```python
from build123d import *

# Parameters (mm, degrees)
F0_R     = 6
F1_DEPTH = 3.7
F2_R     = 1.44999
F4_DEPTH = 14
F5_R     = 1


# Not quite as in the source:
# - a fillet or chamfer is up to 0.001 mm smaller than in the source, because OpenCascade refuses the exact size


with BuildPart() as f1:
    # F0 (on Top) → F1 (new body)
    with BuildSketch(Plane.XY):
        with BuildLine():
            ThreePointArc((6.8481749394, -1.45), (6.9619402675, -0.7289634506), (7, 0))
            ThreePointArc((7, 0), (6.9619402675, 0.7289634506), (6.8481749394, 1.45))
            ThreePointArc((6.8481749394, 1.45), (4.9497474683, 4.9497474683), (1.45, 6.8481749394))
            ThreePointArc((1.45, 6.8481749394), (0.7289634506, 6.9619402675), (0, 7))
            ThreePointArc((0, 7), (-0.7289634506, 6.9619402675), (-1.45, 6.8481749394))
            ThreePointArc((-1.45, 6.8481749394), (-4.9497474683, 4.9497474683), (-6.8481749394, 1.45))
            ThreePointArc((-6.8481749394, 1.45), (-6.9619402675, 0.7289634506), (-7, 0))
            ThreePointArc((-7, 0), (-6.9619402675, -0.7289634506), (-6.8481749394, -1.45))
            ThreePointArc((-6.8481749394, -1.45), (-4.9497474683, -4.9497474683), (-1.45, -6.8481749394))
            ThreePointArc((-1.45, -6.8481749394), (-0.7289634506, -6.9619402675), (0, -7))
            ThreePointArc((0, -7), (0.7289634506, -6.9619402675), (1.45, -6.8481749394))
            ThreePointArc((1.45, -6.8481749394), (4.9497474683, -4.9497474683), (6.8481749394, -1.45))
        make_face()
        Circle(F0_R, mode=Mode.SUBTRACT)
        with BuildLine():
            Line((23.2, 0), (7, 0))
            ThreePointArc((7, 0), (6.9619402675, -0.7289634506), (6.8481749394, -1.45))
            Line((6.8481749394, -1.45), (23.2, -1.45))
            Line((23.2, -1.45), (23.2, 0))
        make_face()
        with BuildLine():
            ThreePointArc((6.8481749394, 1.45), (6.9619402675, 0.7289634506), (7, 0))
            Line((7, 0), (23.2, 0))
            Line((23.2, 0), (23.2, 1.45))
            Line((23.2, 1.45), (6.8481749394, 1.45))
        make_face()
        with BuildLine():
            ThreePointArc((0, 7), (0.7289634506, 6.9619402675), (1.45, 6.8481749394))
            Line((1.45, 6.8481749394), (1.45, 23.2))
            Line((1.45, 23.2), (0, 23.2))
            Line((0, 23.2), (0, 7))
        make_face()
        with BuildLine():
            Line((1.45, -23.2), (1.45, -6.8481749394))
            ThreePointArc((1.45, -6.8481749394), (0.7289634506, -6.9619402675), (0, -7))
            Line((0, -7), (0, -23.2))
            Line((0, -23.2), (1.45, -23.2))
        make_face()
        with BuildLine():
            ThreePointArc((-1.45, 6.8481749394), (-0.7289634506, 6.9619402675), (0, 7))
            Line((0, 7), (0, 23.2))
            Line((0, 23.2), (-1.45, 23.2))
            Line((-1.45, 23.2), (-1.45, 6.8481749394))
        make_face()
        with BuildLine():
            Line((0, -23.2), (0, -7))
            ThreePointArc((0, -7), (-0.7289634506, -6.9619402675), (-1.45, -6.8481749394))
            Line((-1.45, -6.8481749394), (-1.45, -23.2))
            Line((-1.45, -23.2), (0, -23.2))
        make_face()
        with BuildLine():
            ThreePointArc((-7, 0), (-6.9619402675, 0.7289634506), (-6.8481749394, 1.45))
            Line((-6.8481749394, 1.45), (-23.2, 1.45))
            Line((-23.2, 1.45), (-23.2, 0))
            Line((-23.2, 0), (-7, 0))
        make_face()
        with BuildLine():
            Line((-23.2, -1.45), (-6.8481749394, -1.45))
            ThreePointArc((-6.8481749394, -1.45), (-6.9619402675, -0.7289634506), (-7, 0))
            Line((-7, 0), (-23.2, 0))
            Line((-23.2, 0), (-23.2, -1.45))
        make_face()
    extrude(amount=F1_DEPTH)

    # F2 (radius 1.45 in the source; OpenCascade refuses exactly that, so slightly less here)
    f2_edges = [f1.edges().sort_by_distance(p)[0] for p in [
        (1.45, 15.024087, 0),
        (15.024087, 1.45, 0),
        (15.024087, -1.45, 0),
        (1.45, -15.024087, 0),
        (-1.45, -15.024087, 0),
        (-15.024087, -1.45, 0),
        (-15.024087, 1.45, 0),
        (-1.45, 15.024087, 0),
    ]]
    fillet(f2_edges, radius=F2_R)

    # F3 (on face) → F4 (join)
    with BuildSketch(Plane.XY.offset(3.7)):
        with BuildLine():
            Line((18.4430881362, 1.45), (18.4430881362, -1.45))
            ThreePointArc((18.4430881362, -1.45), (18.5, 0), (18.4430881362, 1.45))
        make_face()
        with BuildLine():
            Line((6.8481749394, -1.45), (18.4430881362, -1.45))
            Line((18.4430881362, -1.45), (18.4430881362, 1.45))
            Line((18.4430881362, 1.45), (6.8481749394, 1.45))
            ThreePointArc((6.8481749394, 1.45), (7, 0), (6.8481749394, -1.45))
        make_face()
        with BuildLine():
            ThreePointArc((-18.4430881362, 1.45), (-18.5, 0), (-18.4430881362, -1.45))
            Line((-18.4430881362, -1.45), (-18.4430881362, 1.45))
        make_face()
        with BuildLine():
            Line((-18.4430881362, 1.45), (-18.4430881362, -1.45))
            Line((-18.4430881362, -1.45), (-6.8481749394, -1.45))
            ThreePointArc((-6.8481749394, -1.45), (-7, 0), (-6.8481749394, 1.45))
            Line((-6.8481749394, 1.45), (-18.4430881362, 1.45))
        make_face()
        with BuildLine():
            ThreePointArc((-1.45, -18.4430881362), (0, -18.5), (1.45, -18.4430881362))
            Line((1.45, -18.4430881362), (-1.45, -18.4430881362))
        make_face()
        with BuildLine():
            Line((-1.45, -18.4430881362), (1.45, -18.4430881362))
            Line((1.45, -18.4430881362), (1.45, -6.8481749394))
            ThreePointArc((1.45, -6.8481749394), (0, -7), (-1.45, -6.8481749394))
            Line((-1.45, -6.8481749394), (-1.45, -18.4430881362))
        make_face()
        with BuildLine():
            Line((1.45, 6.8481749394), (1.45, 18.4430881362))
            Line((1.45, 18.4430881362), (-1.45, 18.4430881362))
            Line((-1.45, 18.4430881362), (-1.45, 6.8481749394))
            ThreePointArc((-1.45, 6.8481749394), (0, 7), (1.45, 6.8481749394))
        make_face()
        with BuildLine():
            Line((-1.45, 18.4430881362), (1.45, 18.4430881362))
            ThreePointArc((1.45, 18.4430881362), (0, 18.5), (-1.45, 18.4430881362))
        make_face()
    extrude(amount=F4_DEPTH)

    # F5
    f5_edges = [f1.edges().sort_by_distance(p)[0] for p in [
        (12.645632, 1.45, 17.7),
        (18.443088, 1.45, 10.7),
        (20.821544, 1.45, 3.7),
        (20.821544, -1.45, 3.7),
        (18.443088, -1.45, 10.7),
        (12.645632, -1.45, 17.7),
        (1.45, 12.645632, 17.7),
        (-1.45, 12.645632, 17.7),
        (1.45, 18.443088, 10.7),
        (-1.45, 18.443088, 10.7),
        (1.45, 20.821544, 3.7),
        (-1.45, 20.821544, 3.7),
        (0, 18.5, 3.7),
        (-18.443088, 1.45, 10.7),
        (-18.443088, -1.45, 10.7),
        (-20.821544, 1.45, 3.7),
        (-1.45, -18.443088, 10.7),
        (1.45, -18.443088, 10.7),
        (-1.45, -20.821544, 3.7),
        (1.45, -20.821544, 3.7),
        (-20.821544, -1.45, 3.7),
        (-12.645632, 1.45, 17.7),
        (-12.645632, -1.45, 17.7),
        (-1.45, -12.645632, 17.7),
        (1.45, -12.645632, 17.7),
        (-1.45, -6.848175, 10.7),
        (1.45, -6.848175, 10.7),
        (6.848175, -1.45, 10.7),
        (6.848175, 1.45, 10.7),
        (1.45, 6.848175, 10.7),
        (-1.45, 6.848175, 10.7),
        (-6.848175, 1.45, 10.7),
        (-6.848175, -1.45, 10.7),
    ]]
    fillet(f5_edges, radius=F5_R)


solid = f1.part
```
Geometry check sheet. Reference: the model listing, model coordinates, mm. A direction names the side the tool comes from. Round coordinates to 2 decimals unless told otherwise and drop trailing zeros. Loops run counter-clockwise (first coordinate to the right, second up) from the corner with the lowest first, then second, coordinate; pieces in that order, holes last. Notation, with made-up numbers: M 81,17 L 130,17 A9 ccw 130,31 Z; hole C 30,-3 d10. An arc over 180 degrees is marked long. Return JSON: item names as keys, results as strings. Group by question number.
(1) Mould release check, pull along X, two halves, no side actions. Record for faces 4 (the face through (4.9, -5, 1.8)), 5 (the face through (7.268, -1.145, 10.798)), 6 (the face through (13, -1.45, 9)): pulls with the +X half, pulls with the -X half, needs draft (parallel to the pull), parting line crosses it, or undercut.
(2) Section check B-B, the plane y = -4. Enter the section's corners in (x, z).
(3) Section check A-A, the plane z = 13. Give the number of separate pieces and of enclosed holes in the cut face, and give its area (3 significant figures).
(4) Go/stop test with flat-tipped pins: pin 1 (1 mm diameter, centred on x = 0, y = -21, fed in from +Z); pin 2 (6 mm diameter, centred on x = -15.5, z = 6, fed in from -Y); pin 3 (7.5 mm diameter, centred on y = -14.5, z = 9.5, fed in from +X). Record where each tip stops, or that it passes through.
(5) Scan lines: line 1 along Y through (x, z) = (0, 0.8); line 2 along X through (y, z) = (16, 6.5). Record each from-to range of solid material in increasing order. Write a range as [from, to].
(6) Set-up check for faces 1 (the face through (-2, -6, 3.7)), 2 (the face through (-14.9, -1, 0.4)), 3 (the face through (-13, -1.45, 9)): record each of +Z, -Z, +X, -X, +Y, -Y from which the full face is reachable in a straight line by a thin tool's end or side.
Data:
{
 "1": {"face 4": "pulls with the +X half", "face 5": "undercut", "face 6": "needs draft"},
 "2": {"outline": "M -5.74,0 L -4.47,0 L -4.47,3.7 L -5.74,3.7 Z; M 4.47,0 L 5.74,0 L 5.74,3.7 L 4.47,3.7 Z"},
 "3": {"separate pieces": "4", "enclosed holes": "0", "area": "130 mm²"},
 "4": {"pin 1": "z = 3.7", "pin 2": "y = -1.45", "pin 3": "x = 1.45"},
 "5": {"line 1": "[-23.2, -6], [6, 23.2]", "line 2": "[-1.45, 1.45]"},
 "6": {"face 1": "+Z", "face 2": "-Z, -X, -Y", "face 3": "+Z, -Z, -X, -Y"}
}
